For this review, use the dimensioned drawing (mm, ordinates from the lowest corner) and the shaded views. Coordinates: 2 decimals unless noted, no trailing zeros. Write each loop counter-clockwise with the first axis right and the second up, starting at its lowest first coordinate (ties: lowest second). Pieces come first, ordered by that corner, then holes. Notation, with made-up numbers: M 89,9.25 L 131,9.25 A30 ccw 131,45.25 Z; hole C 23,49.5 d10. An arc over 180 degrees is marked long. One line per question, with ' | ' between items.
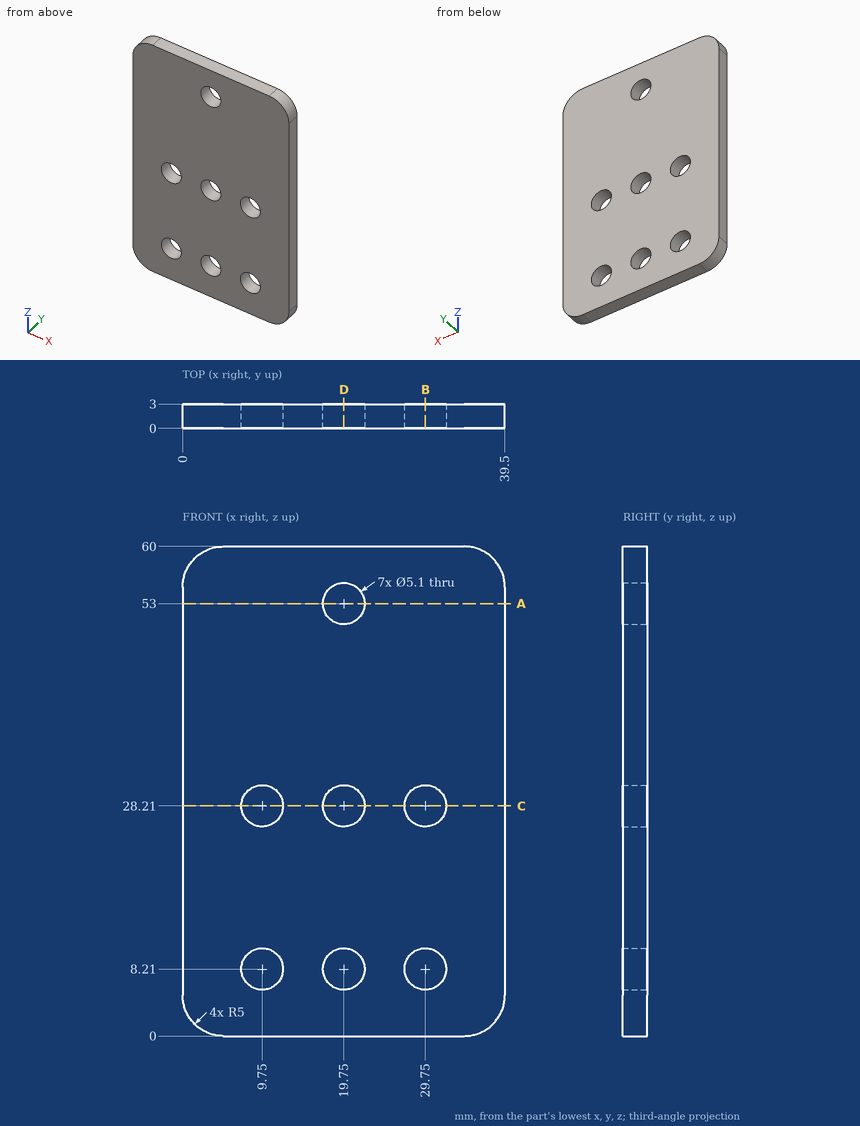
1) To check wall thickness, follow line 1 along Z through (x, y) = (29.75, 1.1); line 2 along X through (y, z) = (1.95, 8.21); line 3 along Z through (x, y) = (19.5, 1.95). State the ranges of each line that lie inside material, in increasing order. Write a range as [from, to].
Responses:
line 1: [0, 5.66], [10.76, 25.66], [30.76, 60] | line 2: [0, 7.2], [12.3, 17.2], [22.3, 27.2], [32.3, 39.5] | line 3: [0, 5.67], [10.75, 25.67], [30.75, 50.46], [55.54, 60]
2) We need section D-D on x = 19.75. State the section outline as (y, z) points, then the cut area to 3 significant figures.
Responses:
outline: M 0,0 L 3,0 L 3,5.66 L 0,5.66 Z; M 0,10.76 L 3,10.76 L 3,25.66 L 0,25.66 Z; M 0,30.76 L 3,30.76 L 3,50.45 L 0,50.45 Z; M 0,55.55 L 3,55.55 L 3,60 L 0,60 Z | area: 134 mm^2
3) We need section B-B on x = 29.75. State the section outline as (y, z) points.
Responses:
outline: M 0,0 L 3,0 L 3,5.66 L 0,5.66 Z; M 0,10.76 L 3,10.76 L 3,25.66 L 0,25.66 Z; M 0,30.76 L 3,30.76 L 3,60 L 0,60 Z
4) Insertion check: pin 1 Ø6 at (x, z) = (19.75, 8.21) entering from +Y; pin 2 Ø4.5 at (x, z) = (19.75, 53) entering from -Y. Each pin has a flat end and moves straight along its axis. Give the tip position at first contact, or say it passes through.
Responses:
pin 1: y = 3 | pin 2: through
5) We need section A-A on z = 53. State the section outline as (x, y) points, then the cut area to 3 significant figures.
Responses:
outline: M 0,0 L 17.2,0 L 17.2,3 L 0,3 Z; M 22.3,0 L 39.5,0 L 39.5,3 L 22.3,3 Z | area: 103 mm^2
6) We need section C-C on z = 28.21. State the section outline as (x, y) points.
Responses:
outline: M 0,0 L 7.2,0 L 7.2,3 L 0,3 Z; M 12.3,0 L 17.2,0 L 17.2,3 L 12.3,3 Z; M 22.3,0 L 27.2,0 L 27.2,3 L 22.3,3 Z; M 32.3,0 L 39.5,0 L 39.5,3 L 32.3,3 Z
